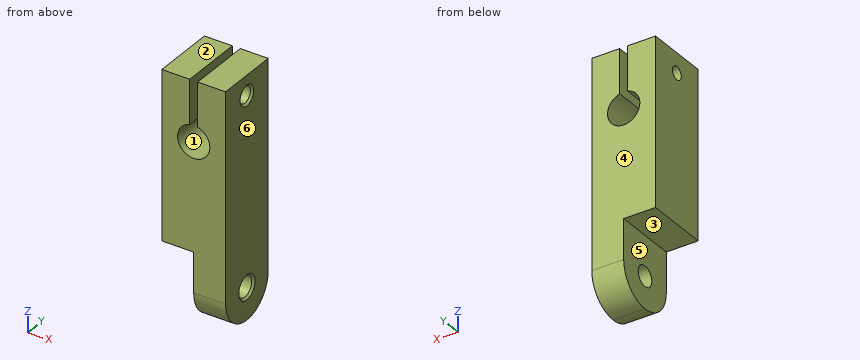
from build123d import *

# Parameters (mm, degrees)
SKETCH1_W                                   = 16
SKETCH1_H                                   = 16
BASE_DEPTH                                  = 60
SKETCH2_R                                   = 4.05
INDICATORHOLE_DEPTH                         = 17
INDICATORMOUNT_REACH                        = 18
SKETCH3_R                                   = 2.05
CHAMFERINDICATORMOUNT_SIZE                  = 0.5
M4X0_7_TAPPED_HOLE_FOR_INDICATORSCREW_D     = 3.3
M4X0_7_TAPPED_HOLE_FOR_INDICATORSCREW_DEPTH = 7.908579979
M4X0_7_TAPPED_HOLE_FOR_INDICATORSCREW_TIP   = 0.991420021
SKETCH6_R                                   = 8
SLOTFORANOTHERPART_DEPTH                    = 9
CHAMFERFORSLOT_DEPTH                        = 9
SKETCH7_R                                   = 2.55
SCREWHOLEFORSLOT_DEPTH                      = 17
CHAMFERFORSCREWSLOT_SIZE                    = 0.5


with BuildPart() as part:
    # Sketch1 → Base (new body)
    with BuildSketch(Plane.XY):
        Rectangle(SKETCH1_W, SKETCH1_H)
    extrude(amount=BASE_DEPTH)

    # Sketch2 → IndicatorHole (cut, through all)
    with BuildSketch(Plane(origin=(0, 8, 0), x_dir=(1, 0, 0), z_dir=(0, 1, 0))):
        with Locations((0, -45)):
            Circle(SKETCH2_R)
        with BuildLine():
            Line((-1, -48.924601891), (-1, -60))
            Line((-1, -60), (1, -60))
            Line((1, -60), (1, -48.924601891))
            ThreePointArc((1, -48.924601891), (0, -49.05), (-1, -48.924601891))
        make_face()
    extrude(amount=-INDICATORHOLE_DEPTH, mode=Mode.SUBTRACT)

    # Sketch3 → IndicatorMount (cut, up to next)
    with BuildSketch(Plane(origin=(8, 0, 0), x_dir=(0, 0, -1), z_dir=(1, 0, 0)), mode=Mode.PRIVATE) as indicatormount_sk1:
        with Locations((-55, 0)):
            Circle(SKETCH3_R)
    indicatormount_tool1 = extrude(indicatormount_sk1.sketch, amount=-INDICATORMOUNT_REACH, mode=Mode.PRIVATE) & part.part
    add(indicatormount_tool1.solids().sort_by_distance((8, 0, 55))[0], mode=Mode.SUBTRACT)

    # ChamferIndicatorMount
    chamferindicatormount_edges = [part.edges().sort_by_distance(p)[0] for p in [
        (8, 0, 57.05),
    ]]
    chamfer(chamferindicatormount_edges, length=CHAMFERINDICATORMOUNT_SIZE)

    # M4x0.7 Tapped Hole for IndicatorScrew
    with Locations(Plane.ZY.offset(8)):
        with Locations((55, 0)):
            Hole(M4X0_7_TAPPED_HOLE_FOR_INDICATORSCREW_D / 2, depth=M4X0_7_TAPPED_HOLE_FOR_INDICATORSCREW_DEPTH)
            with Locations((0, 0, -(M4X0_7_TAPPED_HOLE_FOR_INDICATORSCREW_DEPTH + M4X0_7_TAPPED_HOLE_FOR_INDICATORSCREW_TIP / 2))):  # 118° drill point
                Cone(0, M4X0_7_TAPPED_HOLE_FOR_INDICATORSCREW_D / 2, M4X0_7_TAPPED_HOLE_FOR_INDICATORSCREW_TIP, mode=Mode.SUBTRACT)

    # Sketch6 → SlotForAnotherPart (cut, through all)
    with BuildSketch(Plane(origin=(0, 0, 0), x_dir=(0, 0, -1), z_dir=(1, 0, 0))):
        with BuildLine():
            Line((-8, 8), (-18, 8))
            Line((-18, 8), (-18, -8))
            Line((-18, -8), (-8, -8))
            ThreePointArc((-8, -8), (-16, 0), (-8, 8))
        make_face()
        with Locations((-8, 0)):
            Circle(SKETCH6_R)
        with BuildLine():
            Line((1.86895154, 8), (-8, 8))
            ThreePointArc((-8, 8), (-2.343145751, 5.656854249), (0, 0))
            ThreePointArc((0, 0), (-2.343145751, -5.656854249), (-8, -8))
            Line((-8, -8), (1.86895154, -8))
            Line((1.86895154, -8), (1.86895154, 8))
        make_face()
    extrude(amount=-SLOTFORANOTHERPART_DEPTH, mode=Mode.SUBTRACT)

    # Sketch6_3 → ChamferForSlot (cut, through all)
    with BuildSketch(Plane(origin=(0, 0, 0), x_dir=(0, 0, -1), z_dir=(1, 0, 0))):
        with BuildLine():
            Line((1.86895154, 8), (-8, 8))
            ThreePointArc((-8, 8), (-2.343145751, 5.656854249), (0, 0))
            ThreePointArc((0, 0), (-2.343145751, -5.656854249), (-8, -8))
            Line((-8, -8), (1.86895154, -8))
            Line((1.86895154, -8), (1.86895154, 8))
        make_face()
    extrude(amount=CHAMFERFORSLOT_DEPTH, mode=Mode.SUBTRACT)

    # Sketch7 → ScrewHoleForSlot (cut, through all)
    with BuildSketch(Plane(origin=(8, 0, 0), x_dir=(0, 0, -1), z_dir=(1, 0, 0))):
        with Locations((-8, 0)):
            Circle(SKETCH7_R)
    extrude(amount=-SCREWHOLEFORSLOT_DEPTH, mode=Mode.SUBTRACT)

    # ChamferForScrewSlot
    chamferforscrewslot_edges = [part.edges().sort_by_distance(p)[0] for p in [
        (8, 0, 10.55),
    ]]
    chamfer(chamferforscrewslot_edges, length=CHAMFERFORSCREWSLOT_SIZE)


solid = part.part
Read the model definition and answer for the solid it produces. Units are mm, in the model's axes. Face numbers are marked on the shaded views. A direction names the side the tool comes from. Give positions to 0.01 mm unless a question says otherwise; leave off trailing zeros. Write each loop counter-clockwise with the first axis right and the second up, starting at its lowest first coordinate (ties: lowest second). Pieces come first, ordered by that corner, then holes. Notation, with made-up numbers: (69, 13.25) - (73, 13.25) arc R31 cw to (73, 40.25) - close; hole circle Ø6 at (89.25, 71). An arc over 180 degrees is marked (long way). Return JSON: item names as keys, results as strings.
Q1. A cutting plane is placed at B-B, the plane z = 55. Determine the outline of the cut face in (x, y), and give its area (3 significant figures).
Reply:
{"outline": "(-8, -8) - (-1, -8) - (-1, -1.65) - (-8, -1.65) - close; (-8, 1.65) - (-1, 1.65) - (-1, 8) - (-8, 8) - close; (1, -8) - (8, -8) - (8, -2.55) - (7.5, -2.05) - (1, -2.05) - close; (1, 2.05) - (7.5, 2.05) - (8, 2.55) - (8, 8) - (1, 8) - close", "area": "172 mm²"}
Q2. For a pull along Z with two mould halves and no side action, classify the marked faces 1, 2, 3 and 4 as released by +Z, released by -Z, zero draft, split by the parting line, or undercut.
Reply:
{"face 1": "undercut", "face 2": "released by +Z", "face 3": "released by -Z", "face 4": "zero draft"}
Q3. Given P1, Ø4.5, axis at y = 0, z = 55, coming from the +X side; P2, Ø6, axis at y = 0, z = 8, coming from the -X side; P3, Ø2.5, axis at x = -3.5, y = -2.5, coming from the -Z side, each flat-ended and moving along its own axis, determine where each tip first touches the part or whether it passes through.
Reply:
{"P1": "x = 7.7", "P2": "x = 0", "P3": "z = 18"}
Q4. A cutting plane is placed at A-A, the plane z = 45. Determine the outline of the cut face in (x, y).
Reply:
{"outline": "(-8, -8) - (-4.05, -8) - (-4.05, 8) - (-8, 8) - close; (4.05, -8) - (8, -8) - (8, 8) - (4.05, 8) - close"}
Q5. For the marked faces 5 and 6, determine the directions among +Z, -Z, +X, -X, +Y, -Y from which every point of the face is accessible in a straight line to the end or side of a thin tool.
Reply:
{"face 5": "-Z, -X, +Y, -Y", "face 6": "+Z, -Z, +X, +Y, -Y"}
Q6. Consider line 1 along Y through (x, z) = (5.25, 55); line 2 along Y through (x, z) = (-2.5, 55); line 3 along X through (y, z) = (5.5, 55.5). Determine where each line is inside the solid, lowest interval first. Write a range as [from, to].
Reply:
{"line 1": "[-8, -2.05], [2.05, 8]", "line 2": "[-8, -1.65], [1.65, 8]", "line 3": "[-8, -1], [1, 8]"}
Q7. A cutting plane is placed at C-C, the plane y = -4.5. Determine the outline of the cut face in (x, z), and give its area (3 significant figures).
Reply:
{"outline": "(-8, 18) - (0, 18) - (0, 1.39) - (8, 1.39) - (8, 60) - (1, 60) - (1, 48.92) arc R4.05 cw (long way) to (-1, 48.92) - (-1, 60) - (-8, 60) - close", "area": "731 mm²"}
